```python
from build123d import *

# Parameters (mm, degrees)
SKETCH1_R               = 12.7
BOSS_EXTRUDE1_DEPTH     = 12.7
SKETCH2_R               = 1.905
BOSS_EXTRUDE2_DEPTH     = 3.81
SKETCH3_R               = 6.35
BOSS_EXTRUDE3_DEPTH     = 12.7
SKETCH4_R               = 8.89
BOSS_EXTRUDE4_DEPTH     = 2.54
SKETCH5_R               = 3.175
BOSS_EXTRUDE5_DEPTH     = 21.59
SKETCH6_R               = 1.905
CUT_EXTRUDE1_DEPTH      = 22.5900001
CUT_EXTRUDE1_DEPTH_BACK = 22.5900001


with BuildPart() as part:
    # Sketch1 → Boss-Extrude1 (new body, symmetric)
    with BuildSketch(Plane.XY):
        Circle(SKETCH1_R)
    extrude(amount=BOSS_EXTRUDE1_DEPTH, both=True)

    # Sketch2 → Boss-Extrude2 (add)
    with BuildSketch(Plane(origin=(0, 12.7, 0), x_dir=(1, 0, 0), z_dir=(0, 1, 0))):
        with BuildLine():
            Line((0, 12.7), (0, -12.7))
            Line((0, -12.7), (-11.368596271, -12.7))
            ThreePointArc((-11.368596271, -12.7), (-12.656501603, -12.865969083), (-13.860252421, -13.353031553))
            Line((-13.860252421, -13.353031553), (-29.881257888, -22.370226336))
            ThreePointArc((-29.881257888, -22.370226336), (-34.614455572, -21.562169237), (-34.798, -16.764))
            Line((-34.798, -16.764), (-14.224, 10.668))
            ThreePointArc((-14.224, 10.668), (-12.431845065, 12.16369013), (-10.16, 12.7))
            Line((-10.16, 12.7), (0, 12.7))
        make_face()
        with Locations((-31.75, -19.05)):
            Circle(SKETCH2_R, mode=Mode.SUBTRACT)
    extrude(amount=-BOSS_EXTRUDE2_DEPTH)

    # Sketch3 → Boss-Extrude3 (add)
    with BuildSketch(Plane(origin=(0, 0, -12.7), x_dir=(-1, 0, 0), z_dir=(0, 0, -1))):
        Circle(SKETCH3_R)
    extrude(amount=BOSS_EXTRUDE3_DEPTH)

    # Sketch4 → Boss-Extrude4 (add)
    with BuildSketch(Plane(origin=(0, 0, -25.4), x_dir=(-1, 0, 0), z_dir=(0, 0, -1))):
        Circle(SKETCH4_R)
    extrude(amount=BOSS_EXTRUDE4_DEPTH)

    # Sketch5 → Boss-Extrude5 (add, symmetric)
    with BuildSketch(Plane(origin=(0, 0, 0), x_dir=(1, 0, 0), z_dir=(0, 1, 0))):
        with Locations((0, -6.35)):
            Circle(SKETCH5_R)
    extrude(amount=BOSS_EXTRUDE5_DEPTH, both=True)

    # Sketch6 → Cut-Extrude1 (cut, two sides)
    with BuildSketch(Plane(origin=(0, 0, 0), x_dir=(1, 0, 0), z_dir=(0, 1, 0))) as cut_extrude1_sk:
        with Locations((0, -6.35)):
            Circle(SKETCH6_R)
    extrude(amount=CUT_EXTRUDE1_DEPTH, mode=Mode.SUBTRACT)
    extrude(cut_extrude1_sk.sketch, amount=-CUT_EXTRUDE1_DEPTH_BACK, mode=Mode.SUBTRACT)


solid = part.part
```
For this review, take the finished solid that the model builds, in its own axes (mm). A direction names the side the tool comes from. Round coordinates to 2 decimals unless told otherwise and drop trailing zeros. Write each loop counter-clockwise with the first axis right and the second up, starting at its lowest first coordinate (ties: lowest second). Pieces come first, ordered by that corner, then holes. Notation, with made-up numbers: (45.5, -23) -> (57.5, -23) arc R34 ccw to (57.5, 7) -> close; hole circle Ø7 at (-3.5, 45.5). An arc over 180 degrees is marked (long way). Use one line per item in the form item = value.
1) Tool access review of faces 5 (the cylindrical face through (1.93, -8.68, -26.65)), 6 (the flat face through (-19, 8.89, 5)), 7 (the flat face through (-3, 6, -12.7)), 8 (the cylindrical face through (-0.69, -16.88, 9.45)): name each direction out of +Z, -Z, +X, -X, +Y, -Y from which nothing blocks a thin tool from reaching the whole face with its end or side.
Found:
face_5 = -Z
face_6 = +Z, -Z, -X
face_7 = none
face_8 = -Y
2) Take a section at C-C, the plane z = 19.05. Write out the cut boundary in (x, y) (3 decimals).
Found:
outline = (-35.56, 8.89) -> (-33.655, 8.89) -> (-33.655, 12.7) -> (-35.56, 12.7) -> close; (-29.845, 8.89) -> (-23.982, 8.89) -> (-23.982, 12.7) -> (-29.845, 12.7) -> close
3) Mouldability with a two-part tool opening along Z and no side actions: class faces 1 (the flat face through (-14, 12.7, 5)), 2 (the cylindrical face through (-12.46, 10.82, -12.15)), 3 (the cylindrical face through (-0.69, 17.01, 9.45)), 4 (the cylindrical face through (-0.41, 0.3, 8.21)) as +Z half, -Z half, draft (parallel to the pull), parting line (faces both ways), or undercut.
Found:
face_1 = draft
face_2 = -Z half
face_3 = parting line
face_4 = undercut
4) Take a section at A-A, the plane x = -31.75. Write out the cut boundary in (y, z) (3 decimals), and give its area (3 significant figures).
Found:
outline = (8.89, 12.7) -> (12.7, 12.7) -> (12.7, 17.145) -> (8.89, 17.145) -> close; (8.89, 20.955) -> (12.7, 20.955) -> (12.7, 22.86) -> (8.89, 22.86) -> close
area = 24.2 mm2
5) Take a section at D-D, the plane y = 10.5. Write out the cut boundary in (x, z) (3 decimals), and give its area (3 significant figures).
Found:
outline = (-34.798, 16.764) -> (-14.224, -10.668) arc R5.08 ccw to (-10.16, -12.7) -> (7.144, -12.7) -> (7.144, 12.7) -> (-11.369, 12.7) arc R5.08 cw to (-13.86, 13.353) -> (-29.881, 22.37) arc R3.81 ccw to start; hole circle Ø3.81 at (-31.75, 19.05); hole circle Ø3.81 at (0, 6.35)
area = 850 mm2
6) Clearance check with flat-ended pins moving along their axes: pin 1 (4.5 mm diameter, centred on x = -31.75, z = 19.05, fed in from -Y); pin 2 (4 mm diameter, centred on x = -2, y = -2, fed in from +Z); pin 3 (8 mm diameter, centred on y = -3.5, z = 4, fed in from -X). State where each tip first meets the part, or that it passes through.
Found:
pin_1 = 8.89
pin_2 = 12.7
pin_3 = -12.7
7) To check wall thickness, follow L1, parallel to Z at x = 0, y = 8.5 (3 decimals); L2, parallel to Z at x = -3.5, y = -8; L3, parallel to Z at x = -31.75, y = 10.35 (3 decimals). State the ranges of each line that lie inside material, in increasing order. Write a range as from..to.
Found:
L1 = -27.94..-25.4, -12.7..4.445, 8.255..12.7
L2 = -27.94..-25.4, -12.7..12.7
L3 = 12.7..17.145, 20.955..22.86
8) Take a section at B-B, the plane y = 0. Write out the cut boundary in (x, z) (3 decimals).
Found:
outline = (-12.7, -12.7) -> (-6.35, -12.7) -> (-6.35, -25.4) -> (-8.89, -25.4) -> (-8.89, -27.94) -> (8.89, -27.94) -> (8.89, -25.4) -> (6.35, -25.4) -> (6.35, -12.7) -> (12.7, -12.7) -> (12.7, 12.7) -> (-12.7, 12.7) -> close; hole circle Ø3.81 at (0, 6.35)
